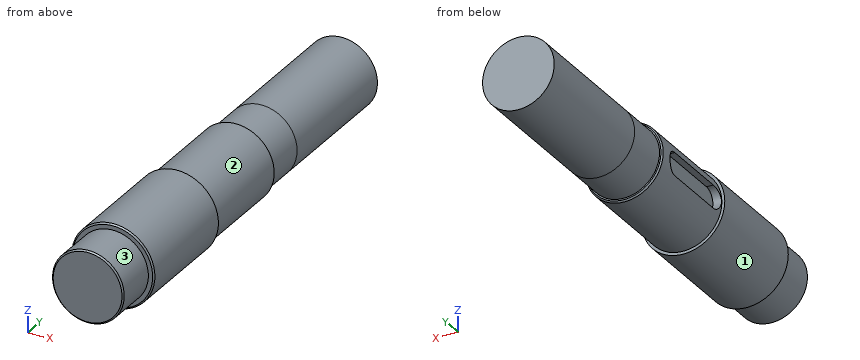
from build123d import *

# Parameters (mm, degrees)
CHAMFER1_SIZE       = 1
CUT_EXTRUDE1_DEPTH  = 6
SKETCH3_R           = 25
BOSS_EXTRUDE1_DEPTH = 100


with BuildPart() as part:
    # Sketch1 → Revolve1 (revolve)
    with BuildSketch(Plane.XY):
        Polygon((0, 87.391304348), (0, -128.608695652), (-25, -128.608695652), (-25, -97.608695652), (-29, -97.608695652), (-29, -17.608695652), (-27, -17.608695652), (-27, 56.391304348), (-25, 56.391304348), (-25, 87.391304348), align=None)
    revolve(axis=Axis((0, 87.391304348, 0), (0, -1, 0)))

    # Chamfer1
    chamfer1_edges = [part.edges().sort_by_distance(p)[0] for p in [
        (27, 56.391304348, 0),
        (25, -128.608695652, 0),
        (29, -97.608695652, 0),
    ]]
    chamfer(chamfer1_edges, length=CHAMFER1_SIZE)

    # Sketch2 → Cut-Extrude1 (cut)
    with BuildSketch(Plane.ZY.offset(27)):
        with BuildLine():
            Line((-8, -9.088294883), (-8, 38.911705117))
            ThreePointArc((-8, 38.911705117), (0, 46.911705117), (8, 38.911705117))
            Line((8, 38.911705117), (8, -9.088294883))
            ThreePointArc((8, -9.088294883), (0, -17.088294883), (-8, -9.088294883))
        make_face()
    extrude(amount=-CUT_EXTRUDE1_DEPTH, mode=Mode.SUBTRACT)

    # Sketch3 → Boss-Extrude1 (add)
    with BuildSketch(Plane(origin=(0, 87.391304348, 0), x_dir=(1, 0, 0), z_dir=(0, 1, 0))):
        Circle(SKETCH3_R)
    extrude(amount=BOSS_EXTRUDE1_DEPTH)


solid = part.part
The model under review builds one solid part; all positions refer to its coordinate system, in mm. Face numbers are marked on the shaded views. A direction names the side the tool comes from. Coordinates: 2 decimals unless noted, no trailing zeros. Loops run counter-clockwise (first coordinate to the right, second up) from the corner with the lowest first, then second, coordinate; pieces in that order, holes last.
(1) Consider section C-C, the plane y = 118. Give the boundary of the cut face in (x, z).
Determined:
outline: circle Ø50 at (0, 0)
(2) Tool access review of the marked faces 1, 2 and 3: name each direction out of +Z, -Z, +X, -X, +Y, -Y from which nothing blocks a thin tool from reaching the whole face with its end or side.
Determined:
face 1: +Y, -Y
face 2: +Y
face 3: -Y
(3) Consider section B-B, the plane x = 0. Give the boundary of the cut face in (y, z).
Determined:
outline: (-128.61, -24) - (-127.61, -25) - (-97.61, -25) - (-97.61, -28) - (-96.61, -29) - (-17.61, -29) - (-17.61, -27) - (55.39, -27) - (56.39, -26) - (56.39, -25) - (187.39, -25) - (187.39, 25) - (56.39, 25) - (56.39, 26) - (55.39, 27) - (-17.61, 27) - (-17.61, 29) - (-96.61, 29) - (-97.61, 28) - (-97.61, 25) - (-127.61, 25) - (-128.61, 24) - close
(4) Consider section A-A, the plane z = 0. Give the boundary of the cut face in (x, y), plus the area to 3 significant figures.
Determined:
outline: (-29, -96.61) - (-28, -97.61) - (-25, -97.61) - (-25, -127.61) - (-24, -128.61) - (24, -128.61) - (25, -127.61) - (25, -97.61) - (28, -97.61) - (29, -96.61) - (29, -17.61) - (27, -17.61) - (27, 55.39) - (26, 56.39) - (25, 56.39) - (25, 187.39) - (-25, 187.39) - (-25, 56.39) - (-26, 56.39) - (-27, 55.39) - (-27, 46.91) - (-21, 46.91) - (-21, -17.09) - (-27, -17.09) - (-27, -17.61) - (-29, -17.61) - close
area: 16,300 mm2
(5) Wall thickness on L1, parallel to Y at x = 17, z = -17; L2, parallel to Y at x = -23.5, z = -7; L3, parallel to Z at x = 17, y = -108: over which ranges is each line inside the solid? List them lowest first.
Determined:
L1: y = -128.57 to 187.39
L2: y = -128.09 to -12.96, 42.78 to 187.39
L3: z = -18.33 to 18.33
(6) Insertion check: P1, Ø6, axis at x = -11.5, y = -53.5, coming from the -Z side; P2, Ø10, axis at x = -18, z = 20, coming from the +Y side; P3, Ø5.5, axis at x = -22.5, y = 11, coming from the -Z side; P4, Ø8, axis at y = 14.5, z = -1, coming from the -X side. Each pin has a flat end and moves straight along its axis. Give the tip position at first contact, or say it passes through.
Determined:
P1: stops at z = -27.73
P2: stops at y = 187.39
P3: stops at z = -18.41
P4: stops at x = -21
